```python
from build123d import *

# Parameters (mm, degrees)
BOSS_EXTRUDE1_DEPTH = 34
SKETCH2_R           = 1.1
CUT_EXTRUDE1_DEPTH  = 4
SKETCH3_R           = 1.25
SKETCH3_R_2         = 0.75
CUT_EXTRUDE2_DEPTH  = 3


with BuildPart() as part:
    # Sketch1 → Boss-Extrude1 (new body)
    with BuildSketch(Plane(origin=(0, 0, 0), x_dir=(0, 0, -1), z_dir=(1, 0, 0))):
        Polygon((0, 0), (6, 0), (6, 35), (3, 35), (3, 2), (0, 2), align=None)
    extrude(amount=BOSS_EXTRUDE1_DEPTH)

    # Sketch2 → Cut-Extrude1 (cut, through all)
    with BuildSketch(Plane.XY.offset(-3)):
        with Locations((23.25, 29.5)):
            Circle(SKETCH2_R)
        with Locations((10.75, 29.5)):
            Circle(SKETCH2_R)
        with Locations((10.75, 8.5)):
            Circle(SKETCH2_R)
        with Locations((23.25, 8.5)):
            Circle(SKETCH2_R)
    extrude(amount=-CUT_EXTRUDE1_DEPTH, mode=Mode.SUBTRACT)

    # Sketch3 → Cut-Extrude2 (cut, through all)
    with BuildSketch(Plane(origin=(0, 2, 0), x_dir=(1, 0, 0), z_dir=(0, 1, 0))):
        with Locations((17, 1.5)):
            Circle(SKETCH3_R)
        with Locations((22, 1.5)):
            Circle(SKETCH3_R_2)
        with Locations((25, 1.5)):
            Circle(SKETCH3_R_2)
        with Locations((12, 1.5)):
            Circle(SKETCH3_R_2)
        with Locations((9, 1.5)):
            Circle(SKETCH3_R_2)
    extrude(amount=-CUT_EXTRUDE2_DEPTH, mode=Mode.SUBTRACT)


solid = part.part
```
Here's how the part is built. I have some questions about the finished solid (model axes, mm). A direction names the side the tool comes from. Coordinates: 2 decimals unless noted, no trailing zeros. Order: outer loops, then holes, each group sorted by start corner. A loop starts at its lowest first (then second) coordinate and runs counter-clockwise, first axis right, second up. Notation, with made-up numbers: M 52.25,12.5 L 89.25,12.5 A25 ccw 89.25,34.5 Z; hole C 68,86 d5. An arc over 180 degrees is marked long. Answer as a JSON object with one key per item and string values. Group by question number.
(1) If we mould it in two halves opening along Z, with no side actions, what happens to faces 1 (the face through (8.25, 1.01, -1.53)), 2 (the face through (17, 17, -6)), 3 (the face through (11.258, 28.524, -4.479))? For each: released by +Z, released by -Z, zero draft, split by the parting line, or undercut.
(2) Which directions (+Z, -Z, +X, -X, +Y, -Y) give clear straight access to the entire face, cutting with the end or side of a thin tool? Please do faces 4 (the face through (22.15, 8.55, -4.48)), 5 (the face through (17, 19, -3)).
(3) For pin 1 (1.4 mm diameter, centred on x = 9, z = -1.5, fed in from +Y); pin 2 (1.5 mm diameter, centred on x = 9, z = -2, fed in from +Y); pin 3 (3 mm diameter, centred on x = 23.25, y = 8.5, fed in from +Z); pin 4 (3 mm diameter, centred on x = 10.75, y = 29.5, fed in from -Z), each with a flat end and sliding along its axis, tell me the tip position at first contact or that it passes through.
(4) I need wall thicknesses on probe 1 along X at (y, z) = (0.4, -1.5); probe 2 along Y at (x, z) = (10.75, -3.95); probe 3 along Z at (x, y) = (25, 1.05). Which ranges of each line are inside material? Lowest first, please.
(5) Suppose I cut it at B-B, the plane z = -1.5. Please give me the cut outline in (x, y), then the cut area to 3 significant figures.
(6) Suppose I cut it at C-C, the plane x = 17. Please give me the cut outline in (y, z), then the cut area to 3 significant figures.
(7) Suppose I cut it at A-A, the plane x = 10.75. Please give me the cut outline in (y, z), then the cut area to 3 significant figures.
(8) Suppose I cut it at D-D, the plane y = 8.5. Please give me the cut outline in (x, z), then the cut area to 3 significant figures.
Values found:
{
 "1": {"face 1": "undercut", "face 2": "released by -Z", "face 3": "zero draft"},
 "2": {"face 4": "+Z, -Z", "face 5": "+Z, +X, -X, +Y"},
 "3": {"pin 1": "passes through", "pin 2": "stops at y = 2", "pin 3": "stops at z = -3", "pin 4": "stops at z = -6"},
 "4": {"probe 1": "x = 0 to 8.25, 9.75 to 11.25, 12.75 to 15.75, 18.25 to 21.25, 22.75 to 24.25, 25.75 to 34", "probe 2": "y = 0 to 7.4, 9.6 to 28.4, 30.6 to 35", "probe 3": "z = -6 to -2.25, -0.75 to 0"},
 "5": {"outline": "M 0,0 L 8.25,0 L 8.25,2 L 0,2 Z; M 9.75,0 L 11.25,0 L 11.25,2 L 9.75,2 Z; M 12.75,0 L 15.75,0 L 15.75,2 L 12.75,2 Z; M 18.25,0 L 21.25,0 L 21.25,2 L 18.25,2 Z; M 22.75,0 L 24.25,0 L 24.25,2 L 22.75,2 Z; M 25.75,0 L 34,0 L 34,2 L 25.75,2 Z", "area": "51.0 mm^2"},
 "6": {"outline": "M 0,-6 L 35,-6 L 35,-3 L 2,-3 L 2,-2.75 L 0,-2.75 Z; M 0,-0.25 L 2,-0.25 L 2,0 L 0,0 Z", "area": "106 mm^2"},
 "7": {"outline": "M 0,-6 L 7.4,-6 L 7.4,-3 L 2,-3 L 2,0 L 0,0 Z; M 9.6,-6 L 28.4,-6 L 28.4,-3 L 9.6,-3 Z; M 30.6,-6 L 35,-6 L 35,-3 L 30.6,-3 Z", "area": "97.8 mm^2"},
 "8": {"outline": "M 0,-6 L 9.65,-6 L 9.65,-3 L 0,-3 Z; M 11.85,-6 L 22.15,-6 L 22.15,-3 L 11.85,-3 Z; M 24.35,-6 L 34,-6 L 34,-3 L 24.35,-3 Z", "area": "88.8 mm^2"}
}
